Drawing for the job (mm, zero at the part's lowest x, y, z). Coordinates: 2 decimals unless noted, no trailing zeros. Loops run counter-clockwise (first coordinate to the right, second up) from the corner with the lowest first, then second, coordinate; pieces in that order, holes last. Notation, with made-up numbers: (4.5, 82.5) - (18.5, 82.5) arc R17 cw to (18.5, 106.5) - close; hole circle Ø5 at (36.25, 50). An arc over 180 degrees is marked (long way). Put each result on its own line as item: value.
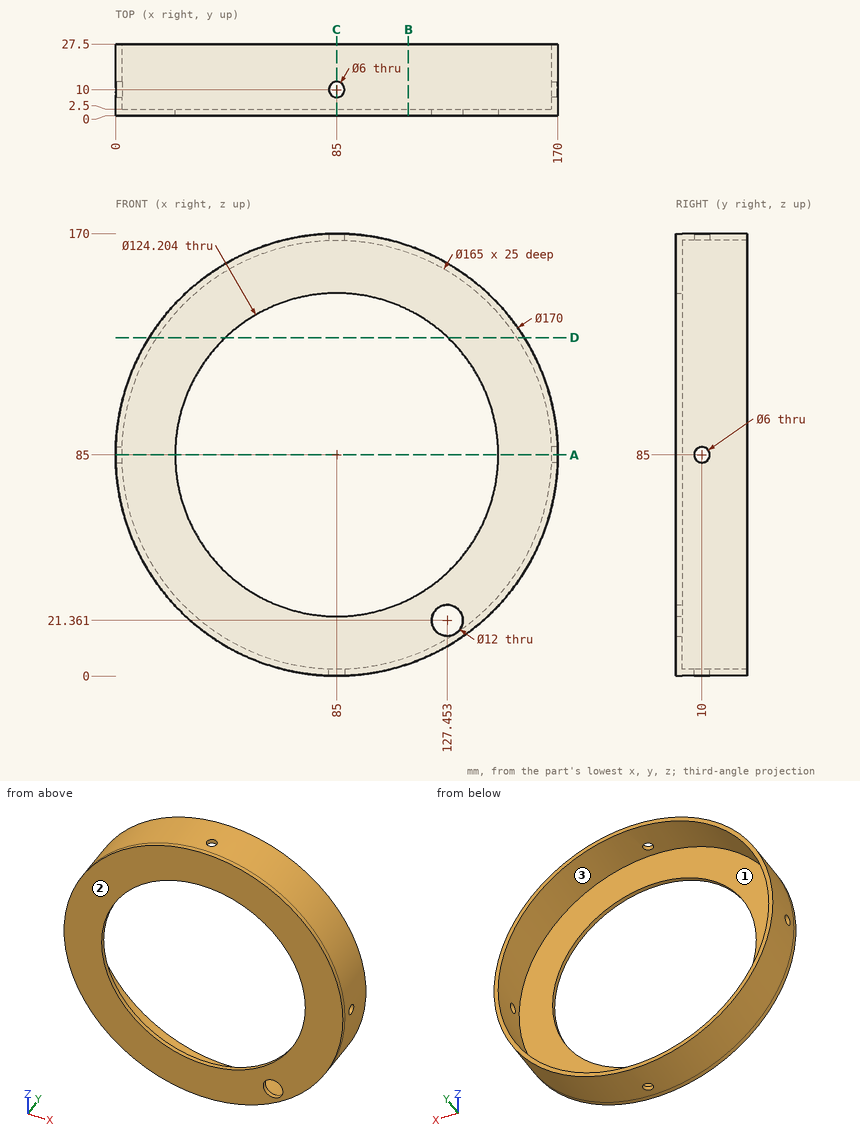
Q1. Slice it at A-A, the plane z = 85. Give the cut face in (x, y).
Determined:
outline: (0, 0) - (22.9, 0) - (22.9, 2.5) - (2.5, 2.5) - (2.5, 7) - (0, 7) - close; (0, 13) - (2.5, 13) - (2.5, 27.5) - (0, 27.5) - close; (147.1, 0) - (170, 0) - (170, 7) - (167.5, 7) - (167.5, 2.5) - (147.1, 2.5) - close; (167.5, 13) - (170, 13) - (170, 27.5) - (167.5, 27.5) - close
Q2. Wall check: L1, parallel to Z at x = 84, y = 24 (1 decimal); L2, parallel to Y at x = 87, z = 159; L3, parallel to Z at x = 122.5, y = 8.75 (1 decimal). Give the ranges that are in metal, low to high. Write a range as from..to.
Determined:
L1: 0..2.5, 167.5..170
L2: 0..2.5
L3: 8.7..11.5, 158.5..161.3
Q3. Pin check, flat tips, straight feed: pin 1 Ø2 at (y, z) = (18.5, 115) entering from +X; pin 2 Ø12 at (y, z) = (7.5, 146) entering from +X; pin 3 Ø5 at (y, z) = (10, 85) entering from -X; pin 4 Ø4 at (y, z) = (14, 91) entering from +X. Stop position of each tip, or through.
Determined:
pin 1: x = 164.9
pin 2: x = 149.81
pin 3: through
pin 4: x = 169.91
Q4. Slice it at B-B, the plane x = 112.5. Give the cut face in (y, z).
Determined:
outline: (0, 4.57) - (27.5, 4.57) - (27.5, 7.22) - (2.5, 7.22) - (2.5, 29.32) - (0, 29.32) - close; (0, 140.68) - (2.5, 140.68) - (2.5, 162.78) - (27.5, 162.78) - (27.5, 165.43) - (0, 165.43) - close
Q5. Slice it at D-D, the plane z = 130. Give the cut face in (x, y), then the cut area to 3 significant figures.
Determined:
outline: (12.89, 0) - (42.2, 0) - (42.2, 2.5) - (15.85, 2.5) - (15.85, 27.5) - (12.89, 27.5) - close; (127.8, 0) - (157.11, 0) - (157.11, 27.5) - (154.15, 27.5) - (154.15, 2.5) - (127.8, 2.5) - close
area: 295 mm2
Q6. Slice it at C-C, the plane x = 85. Give the cut face in (y, z).
Determined:
outline: (0, 0) - (7, 0) - (7, 2.5) - (2.5, 2.5) - (2.5, 22.9) - (0, 22.9) - close; (0, 147.1) - (2.5, 147.1) - (2.5, 167.5) - (7, 167.5) - (7, 170) - (0, 170) - close; (13, 0) - (27.5, 0) - (27.5, 2.5) - (13, 2.5) - close; (13, 167.5) - (27.5, 167.5) - (27.5, 170) - (13, 170) - close
Q7. Mould opens along X. For the marked faces 1, 2 and 3 say: +X half, -X half, draft (parallel to the pull), parting line (faces both ways), or undercut.
Determined:
face 1: undercut
face 2: draft
face 3: undercut
